Could you check a few things on this model? Use its own coordinates, in mm. Face numbers are marked on the shaded views. A direction names the side the tool comes from. Round coordinates to 2 decimals unless told otherwise and drop trailing zeros. Write each loop counter-clockwise with the first axis right and the second up, starting at its lowest first coordinate (ties: lowest second). Pieces come first, ordered by that corner, then holes. Notation, with made-up numbers: (80, 52.5) - (99, 52.5) arc R13 cw to (99, 59.5) - close; hole circle Ø1 at (29, 13). An arc over 180 degrees is marked (long way). Put each result on its own line as item: value.
from build123d import *

# Parameters (mm, degrees)
SKETCH2_W               = 75.057
SKETCH2_H               = 120.142
BOSS_EXTRUDE1_DEPTH     = 76.2
CUT_EXTRUDE1_REACH      = 106.035
SKETCH6_W               = 65.532
SKETCH6_H               = 110.617
FILLET1_R               = 1.27
CUT_EXTRUDE3_DEPTH      = 148.135748465
CUT_EXTRUDE3_DEPTH_BACK = 148.135748465
SKETCH7_R               = 2.0955


with BuildPart() as part:
    # Sketch2 → Boss-Extrude1 (new body)
    with BuildSketch(Plane(origin=(0, 0, 0), x_dir=(0, 0, -1), z_dir=(1, 0, 0))):
        Rectangle(SKETCH2_W, SKETCH2_H)
    extrude(amount=BOSS_EXTRUDE1_DEPTH)

    # Sketch6 → Cut-Extrude1 (cut, up to next)
    with BuildSketch(Plane.ZY, mode=Mode.PRIVATE) as cut_extrude1_sk1:
        Rectangle(SKETCH6_W, SKETCH6_H)
    cut_extrude1_tool1 = extrude(cut_extrude1_sk1.sketch, amount=-CUT_EXTRUDE1_REACH, mode=Mode.PRIVATE) & part.part
    add(cut_extrude1_tool1.solids().sort_by_distance((0, 0, 0))[0], mode=Mode.SUBTRACT)

    # Fillet1
    fillet1_edges = [part.edges().sort_by_distance(p)[0] for p in [
        (38.1, -60.071, -37.5285),
        (38.1, -60.071, 37.5285),
        (38.1, 60.071, 37.5285),
        (38.1, 60.071, -37.5285),
    ]]
    fillet(fillet1_edges, radius=FILLET1_R)

    # Sketch7 → Cut-Extrude3 (cut, two sides: drawn at the far end of the back side and taken through both)
    with BuildSketch(Plane.XZ.offset(60.071).offset(-CUT_EXTRUDE3_DEPTH_BACK)):
        with Locations(Location((11.43, 18.1864, 0), (0, 0, 270))):
            Circle(SKETCH7_R)
        with Locations(Location((64.77, 18.1864, 0), (0, 0, 270))):
            Circle(SKETCH7_R)
        with Locations(Location((11.43, -16.9799, 0), (0, 0, 270))):
            Circle(SKETCH7_R)
        with Locations(Location((64.77, -16.9799, 0), (0, 0, 270))):
            Circle(SKETCH7_R)
    extrude(amount=CUT_EXTRUDE3_DEPTH + CUT_EXTRUDE3_DEPTH_BACK, mode=Mode.SUBTRACT)


solid = part.part
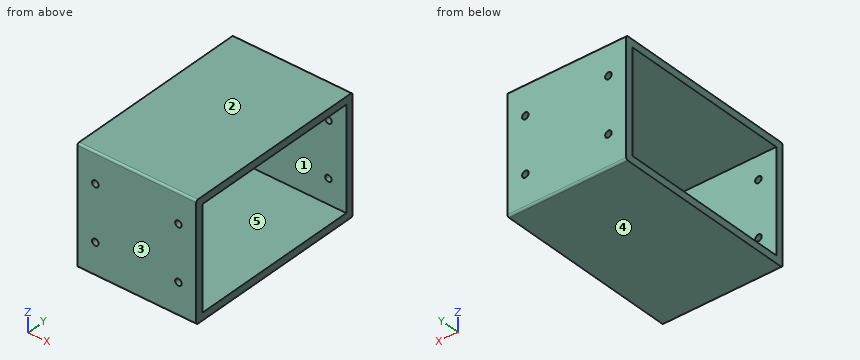
(1) Imagine slicing it at B-B, the plane z = 14. List the corners of the cut face in (x, y) for me.
Values found:
outline: (0, -60.07) - (76.2, -60.07) - (76.2, -55.31) - (0, -55.31) - close; (0, 55.31) - (76.2, 55.31) - (76.2, 60.07) - (0, 60.07) - close
(2) I'm going to push a flat-ended pin straight in: pin 1 (4 mm diameter, centred on x = 11.43, z = 18.19, fed in from -Y). Where does the tip first touch, or does it pass through?
Values found:
pin 1: passes through
(3) If we mould it in two halves opening along Y, with no side actions, what happens to the marked faces 1, 2 and 3? For each: pulls with the +Y half, pulls with the -Y half, needs draft (parallel to the pull), parting line crosses it, or undercut.
Values found:
face 1: undercut
face 2: needs draft
face 3: pulls with the -Y half
(4) Please list where these lines run through material, in increasing order: probe 1 along Z at (x, y) = (64.77, 58.9); probe 2 along Z at (x, y) = (8.5, -26); probe 3 along Y at (x, z) = (58, -3.5). Write a range as from..to.
Values found:
probe 1: z = -37.52..-19.08, -14.88..16.09, 20.28..37.52
probe 2: z = -37.53..-32.77, 32.77..37.53
probe 3: y = -60.07..-55.31, 55.31..60.07
(5) For the marked faces 4 and 5, which set-ups out of +Z, -Z, +X, -X, +Y, -Y let a thin tool reach every point of the face, with its end or its side?
Values found:
face 4: -Z, +X, -X, +Y, -Y
face 5: +X, -X
(6) Imagine slicing it at C-C, the plane y = -49. List the corners of the cut face in (x, z) for me, then the cut area to 3 significant figures.
Values found:
outline: (0, -37.53) - (76.2, -37.53) - (76.2, -32.77) - (0, -32.77) - close; (0, 32.77) - (76.2, 32.77) - (76.2, 37.53) - (0, 37.53) - close
area: 726 mm^2
(7) Imagine slicing it at D-D, the plane x = 53. List the corners of the cut face in (y, z) for me.
Values found:
outline: (-60.07, -36.26) arc R1.27 ccw to (-58.8, -37.53) - (58.8, -37.53) arc R1.27 ccw to (60.07, -36.26) - (60.07, 36.26) arc R1.27 ccw to (58.8, 37.53) - (-58.8, 37.53) arc R1.27 ccw to (-60.07, 36.26) - close; hole (-55.31, -32.77) - (55.31, -32.77) - (55.31, 32.77) - (-55.31, 32.77) - close
(8) Imagine slicing it at A-A, the plane x = 64.77. List the corners of the cut face in (y, z) for me.
Values found:
outline: (-60.07, -36.26) arc R1.27 ccw to (-58.8, -37.53) - (58.8, -37.53) arc R1.27 ccw to (60.07, -36.26) - (60.07, -19.08) - (55.31, -19.08) - (55.31, -32.77) - (-55.31, -32.77) - (-55.31, -19.08) - (-60.07, -19.08) - close; (-60.07, -14.88) - (-55.31, -14.88) - (-55.31, 16.09) - (-60.07, 16.09) - close; (-60.07, 20.28) - (-55.31, 20.28) - (-55.31, 32.77) - (55.31, 32.77) - (55.31, 20.28) - (60.07, 20.28) - (60.07, 36.26) arc R1.27 ccw to (58.8, 37.53) - (-58.8, 37.53) arc R1.27 ccw to (-60.07, 36.26) - close; (55.31, -14.88) - (60.07, -14.88) - (60.07, 16.09) - (55.31, 16.09) - close
